Read the model definition and answer for the solid it produces. Units are mm, in the model's axes. A direction names the side the tool comes from. Give positions to 0.01 mm unless a question says otherwise; leave off trailing zeros. Order: outer loops, then holes, each group sorted by start corner. A loop starts at its lowest first (then second) coordinate and runs counter-clockwise, first axis right, second up. Notation, with made-up numbers: (60, -3) -> (106, -3) arc R18 ccw to (106, 29) -> close; hole circle Ø3 at (68, -19.75). An arc over 180 degrees is marked (long way). One line per item, written item: value. Start each with the question number.
from build123d import *

# Parameters (mm, degrees)
SKETCH1_W               = 50.8
SKETCH1_H               = 25.4
BOSS_EXTRUDE1_DEPTH     = 26.67
SKETCH2_W               = 6.35
SKETCH2_H               = 25.4
BOSS_EXTRUDE2_DEPTH     = 25.4
SKETCH3_W               = 25.4
SKETCH3_H               = 25.4
BOSS_EXTRUDE3_DEPTH     = 25.4
CHAMFER1_SIZE           = 12.7
SKETCH4_R               = 2.413
CUT_EXTRUDE1_DEPTH      = 71.034483649
SKETCH4_4_R             = 4.445
SKETCH4_4_R_2           = 2.413
CUT_EXTRUDE2_DEPTH      = 5.08
CUT_EXTRUDE3_DEPTH      = 29.972
CUT_EXTRUDE3_DEPTH_BACK = 1.27
CUT_EXTRUDE3_START      = -25.4
SKETCH5_R               = 4.445
CHAMFER3_SIZE           = 2.54
FILLET1_R               = 22.86


with BuildPart() as part:
    # Sketch1 → Boss-Extrude1 (new body)
    with BuildSketch(Plane(origin=(0, 0, 0), x_dir=(1, 0, 0), z_dir=(0, 1, 0))):
        with Locations((-38.1, 0)):
            Rectangle(SKETCH1_W, SKETCH1_H)
    extrude(amount=BOSS_EXTRUDE1_DEPTH)



with BuildPart() as body_2:
    # Sketch2 → Boss-Extrude2 (new body)
    with BuildSketch(Plane(origin=(0, 26.67, 0), x_dir=(1, 0, 0), z_dir=(0, 1, 0))):
        with Locations((-9.525, 0)):
            Rectangle(SKETCH2_W, SKETCH2_H)
    extrude(amount=BOSS_EXTRUDE2_DEPTH)


with BuildPart() as part_1:
    add(part.part)

    add(body_2.part)  # Boss-Extrude3 merges body 2
    # Sketch3 → Boss-Extrude3 (add)
    with BuildSketch(Plane(origin=(0, 26.67, 0), x_dir=(1, 0, 0), z_dir=(0, 1, 0))):
        with Locations((-25.4, 0)):
            Rectangle(SKETCH3_W, SKETCH3_H)
    extrude(amount=BOSS_EXTRUDE3_DEPTH)

    # Chamfer1
    chamfer1_edges = [part_1.edges().sort_by_distance(p)[0] for p in [
        (-38.1, 26.67, 0),
    ]]
    chamfer(chamfer1_edges, length=CHAMFER1_SIZE)

    # Sketch4 → Cut-Extrude1 (cut, through all)
    with BuildSketch(Plane(origin=(0, 26.67, 0), x_dir=(1, 0, 0), z_dir=(0, 1, 0))):
        with Locations(Location((-57.15, 0, 0), (0, 0, 270))):
            Circle(SKETCH4_R)
        with Locations(Location((-29.339108581, 0, 0), (0, 0, 270))):
            Circle(SKETCH4_R)
    extrude(amount=-CUT_EXTRUDE1_DEPTH, mode=Mode.SUBTRACT)

    # Sketch4<4> → Cut-Extrude2 (cut)
    # profile 1 of 2: a face of its own
    with BuildSketch(Plane(origin=(0, 26.67, 0), x_dir=(1, 0, 0), z_dir=(0, 1, 0))):
        with Locations(Location((-57.15, 0, 0), (0, 0, 270))):
            Circle(SKETCH4_4_R)
        with Locations(Location((-57.15, 0, 0), (0, 0, 270))):
            Circle(SKETCH4_4_R_2, mode=Mode.SUBTRACT)
    # profile 2 of 2: a face of its own
    with BuildSketch(Plane(origin=(0, 26.67, 0), x_dir=(1, 0, 0), z_dir=(0, 1, 0))):
        with Locations(Location((-29.339108581, 0, 0), (0, 0, 270))):
            Circle(SKETCH4_4_R)
        with Locations(Location((-29.339108581, 0, 0), (0, 0, 270))):
            Circle(SKETCH4_4_R_2, mode=Mode.SUBTRACT)
    extrude(amount=-CUT_EXTRUDE2_DEPTH, mode=Mode.SUBTRACT)

    # Sketch5 → Cut-Extrude3 (cut, two sides: drawn at the far end of the back side and taken through both)
    with BuildSketch(Plane(origin=(0, 52.07, 0), x_dir=(1, 0, 0), z_dir=(0, 1, 0)).offset(CUT_EXTRUDE3_START - CUT_EXTRUDE3_DEPTH_BACK)):
        with Locations(Location((-29.339108581, 0, 0), (0, 0, 270))):
            Circle(SKETCH5_R)
    extrude(amount=CUT_EXTRUDE3_DEPTH + CUT_EXTRUDE3_DEPTH_BACK, mode=Mode.SUBTRACT)

    # Chamfer3
    chamfer3_edges = [part_1.edges().sort_by_distance(p)[0] for p in [
        (-12.7, 13.335, -12.7),
        (-12.7, 13.335, 12.7),
        (-63.5, 13.335, -12.7),
        (-63.5, 13.335, 12.7),
    ]]
    chamfer(chamfer3_edges, length=CHAMFER3_SIZE)

    # Fillet1
    # the kernel refuses this fillet: 22.86 mm, written as the material it takes off along each edge
    with BuildSketch(Plane(origin=(-6.35, 52.07, -69.85), x_dir=(-1, 0, 0), z_dir=(0, 0, 1))) as fillet1_piece_1:
        with BuildLine():
            CenterArc((FILLET1_R, FILLET1_R), FILLET1_R, 180, 90)
            Line((0, FILLET1_R), (0, 0))
            Line((0, 0), (FILLET1_R, 0))
        make_face()
    extrude(amount=139.7, mode=Mode.SUBTRACT)


solid = part_1.part
Item 1: A tool of negligible diameter and unlimited length cuts with its end or side. For faces 4 (the flat face through (-38.1, 46, 0)), 5 (the flat face through (-59, 21.59, 2)), 6 (the flat face through (-12.7, 13, 0)), 7 (the cylindrical face through (-59.506, 10.946, -0.523)), 8 (the flat face through (-13.95, 13.15, -11.41)), from which of +Z, -Z, +X, -X, +Y, -Y can it reach the whole face along a straight path? Write none if from no direction.
Item 2: Flat-ended cylindrical pins translate along their axes: pin 1 (4 mm diameter, centred on x = -17.5, z = 5, fed in from -Y); pin 2 (5.5 mm diameter, centred on x = -57.15, z = 0, fed in from +Y); pin 3 (1.5 mm diameter, centred on y = 16, z = -8, fed in from +X); pin 4 (4 mm diameter, centred on y = 47, z = 4.5, fed in from -X). Find the tip coordinate at first contact, or state that the pin passes through.
Item 3: Find section D-D on z = 0. Write down the section's boundary in (x, y) (3 decimals), then the cut area to 3 significant figures.
Item 4: Find the intervals of material crossed by line 1 (X direction, y = 25.75, z = 0) (3 decimals); line 2 (X direction, y = 12.5, z = 0); line 3 (Y direction, x = -28.5, z = -10.5), in increasing order. Write a range as from..to.
Item 5: Find section B-B on z = 7.75. Write down the section's boundary in (x, y).
Item 6: Find section A-A on x = -57.15. Write down the section's boundary in (y, z) (3 decimals).
Item 7: For a pull along Z with two mould halves and no side action, classify faces 1 (the cylindrical face through (-26.947, 10.946, -0.314)), 2 (the flat face through (-44.54, 32.93, 0.18)), 3 (the flat face through (-13.95, 13.15, 11.41)) as +Z half, -Z half, draft (parallel to the pull), parting line (faces both ways), or undercut.
Item 8: Find section C-C on y = 24.5. Write down the section's boundary in (x, z) (3 decimals).
Checks:
1. face 4: +Z, -Z, -X, +Y
1. face 5: +Y
1. face 6: +Z, -Z, +X, -Y
1. face 7: +Y, -Y
1. face 8: -Z, +X, -Y
2. pin 1: y = 0
2. pin 2: y = 21.59
2. pin 3: x = -12.7
2. pin 4: x = -38.1
3. outline: (-63.5, 0) -> (-59.563, 0) -> (-59.563, 21.59) -> (-61.595, 21.59) -> (-61.595, 26.67) -> (-63.5, 26.67) -> close; (-54.737, 0) -> (-31.752, 0) -> (-31.752, 21.59) -> (-33.784, 21.59) -> (-33.784, 52.07) -> (-38.1, 52.07) -> (-38.1, 39.37) -> (-50.8, 26.67) -> (-52.705, 26.67) -> (-52.705, 21.59) -> (-54.737, 21.59) -> close; (-26.926, 0) -> (-12.7, 0) -> (-12.7, 26.67) -> (-6.35, 26.67) -> (-6.35, 29.21) arc R22.86 ccw to (-24.894, 51.659) -> (-24.894, 21.59) -> (-26.926, 21.59) -> close
3. area: 1,610 mm2
4. line 1: -63.5..-61.595, -52.705..-33.784, -24.894..-12.7
4. line 2: -63.5..-59.56, -54.74..-31.75, -26.93..-12.7
4. line 3: 0..52.06
5. outline: (-63.5, 0) -> (-12.7, 0) -> (-12.7, 26.67) -> (-6.35, 26.67) -> (-6.35, 29.21) arc R22.86 ccw to (-29.21, 52.07) -> (-38.1, 52.07) -> (-38.1, 39.37) -> (-50.8, 26.67) -> (-63.5, 26.67) -> close
6. outline: (0, -12.7) -> (26.67, -12.7) -> (26.67, -4.445) -> (21.59, -4.445) -> (21.59, -2.413) -> (0, -2.413) -> close; (0, 2.413) -> (21.59, 2.413) -> (21.59, 4.445) -> (26.67, 4.445) -> (26.67, 12.7) -> (0, 12.7) -> close
7. face 1: undercut
7. face 2: draft
7. face 3: +Z half
8. outline: (-63.5, -10.16) -> (-60.96, -12.7) -> (-15.24, -12.7) -> (-12.7, -10.16) -> (-12.7, 10.16) -> (-15.24, 12.7) -> (-60.96, 12.7) -> (-63.5, 10.16) -> close; hole circle Ø8.89 at (-57.15, 0); hole circle Ø8.89 at (-29.339, 0)
